Work out the finished part from the listing and answer in its coordinate system (mm). Face numbers are marked on the shaded views. A direction names the side the tool comes from. Round coordinates to 2 decimals unless told otherwise and drop trailing zeros. Order: outer loops, then holes, each group sorted by start corner. A loop starts at its lowest first (then second) coordinate and runs counter-clockwise, first axis right, second up. Notation, with made-up numbers: (-13, -16) - (2, -16) arc R19 ccw to (2, 4) - close; hole circle Ø1 at (33, 82.5). An arc over 180 degrees is marked (long way). Answer in a Markdown table with one row per item.
from build123d import *

# Parameters (mm, degrees)
SKETCH_1_W          = 31.8
SKETCH_1_H          = 7.8
EXTRUDE_2_DEPTH     = 9.6
SKETCH_2_R          = 2.4
EXTRUDE_3_DEPTH     = 1.7
CUT_EXTRUDE_2_DEPTH = 21.144726357
SKETCH_4_R          = 2.5
CUT_EXTRUDE_3_DEPTH = 1.8


with BuildPart() as part:
    # Эскиз1 → Бобышка-Вытянуть2 (new body)
    with BuildSketch(Plane.XY):
        Rectangle(SKETCH_1_W, SKETCH_1_H)
    extrude(amount=EXTRUDE_2_DEPTH)

    # Эскиз2 → Бобышка-Вытянуть3 (add)
    with BuildSketch(Plane(origin=(0, 0, 0), x_dir=(-1, 0, 0), z_dir=(0, 0, -1))):
        with Locations((-12, 0)):
            Circle(SKETCH_2_R)
        with Locations((-4, 0)):
            Circle(SKETCH_2_R)
        with Locations((4, 0)):
            Circle(SKETCH_2_R)
        with Locations((12, 0)):
            Circle(SKETCH_2_R)
    extrude(amount=EXTRUDE_3_DEPTH)

    # Эскиз3 → Вырез-Вытянуть2 (cut, through all)
    with BuildSketch(Plane.XZ.offset(3.9)):
        with BuildLine():
            Line((8, 9.6), (-8, 9.6))
            ThreePointArc((-8, 9.6), (0, 1.6), (8, 9.6))
        make_face()
    extrude(amount=-CUT_EXTRUDE_2_DEPTH, mode=Mode.SUBTRACT)

    # Эскиз4 → Вырез-Вытянуть3 (cut)
    with BuildSketch(Plane.XY.offset(9.6)):
        with Locations((12, 0)):
            Circle(SKETCH_4_R)
        with Locations((-12, 0)):
            Circle(SKETCH_4_R)
    extrude(amount=-CUT_EXTRUDE_3_DEPTH, mode=Mode.SUBTRACT)


solid = part.part
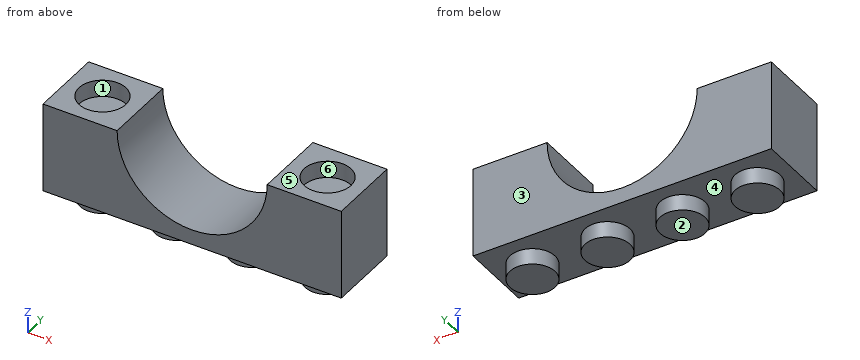
1) Find section C-C, the plane x = -2. Give the vertices of the cut face in (y, z), then the cut area to 3 significant figures.
Filled in:
| item | result |
|---|---|
| outline | (-3.9, 0) - (-1.33, 0) - (-1.33, -1.7) - (1.33, -1.7) - (1.33, 0) - (3.9, 0) - (3.9, 1.85) - (-3.9, 1.85) - close |
| area | 19.0 mm^2 |
2) Find section B-B, the plane z = 3.5. Give the vertices of the cut face in (x, y).
Filled in:
| item | result |
|---|---|
| outline | (-15.9, -3.9) - (-5.18, -3.9) - (-5.18, 3.9) - (-15.9, 3.9) - close; (5.18, -3.9) - (15.9, -3.9) - (15.9, 3.9) - (5.18, 3.9) - close |
3) The mould has two halves that part along Y. Classify the marked faces 1, 2 and 3: released by +Y, released by -Y, zero draft, split by the parting line, or undercut.
Filled in:
| item | result |
|---|---|
| face 1 | undercut |
| face 2 | zero draft |
| face 3 | released by +Y |
4) Which of the six approach directions +Z, -Z, +X, -X, +Y, -Y give full straight-line access (tool end or side, diameter ignored) to the marked faces 4, 5 and 6?
Filled in:
| item | result |
|---|---|
| face 4 | -Z |
| face 5 | +Z, +X, -X, +Y, -Y |
| face 6 | +Z |
5) Find the intervals of material crossed by probe 1 along Y at (x, z) = (-12, 8.45); probe 2 along X at (y, z) = (-0.5, -0.5); probe 3 along Z at (x, y) = (-13.5, -3.5), in increasing order. Write a range as from..to.
Filled in:
| item | result |
|---|---|
| probe 1 | y = -3.9..-2.5, 2.5..3.9 |
| probe 2 | x = -14.35..-9.65, -6.35..-1.65, 1.65..6.35, 9.65..14.35 |
| probe 3 | z = 0..9.6 |
6) Find section D-D, the plane x = 12. Give the vertices of the cut face in (y, z), then the cut area to 3 significant figures.
Filled in:
| item | result |
|---|---|
| outline | (-3.9, 0) - (-2.4, 0) - (-2.4, -1.7) - (2.4, -1.7) - (2.4, 0) - (3.9, 0) - (3.9, 9.6) - (2.5, 9.6) - (2.5, 7.8) - (-2.5, 7.8) - (-2.5, 9.6) - (-3.9, 9.6) - close |
| area | 74.0 mm^2 |
